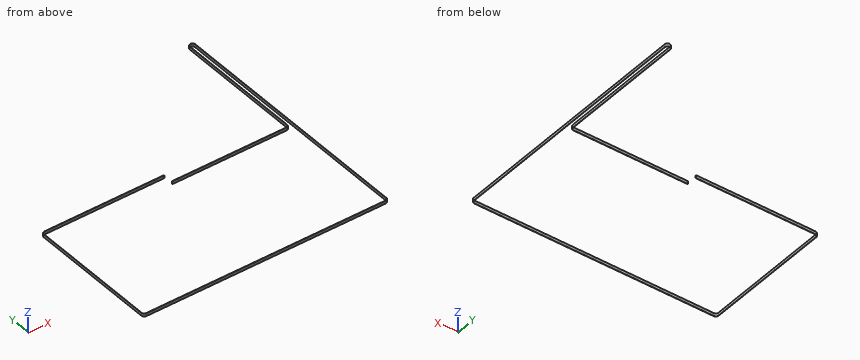
from build123d import *

# Parameters (mm, degrees)
F1_DEPTH = 6


with BuildPart() as f1:
    # F0 (on Top) → F1 (new body)
    with BuildSketch(Plane.XY):
        with BuildLine():
            ThreePointArc((244.655, 259.59), (249.75, 264.685), (254.845, 259.59))
            Line((254.845, 259.59), (254.845, -261.41))
            ThreePointArc((254.845, -261.41), (253.352709, -265.012709), (249.75, -266.505))
            Line((249.75, -266.505), (-249.75, -266.505))
            ThreePointArc((-249.75, -266.505), (-253.352709, -265.012709), (-254.845, -261.41))
            Line((-254.845, -261.41), (-254.845, 5.09))
            Line((-254.845, 5.09), (-255.475, 5.09))
            Line((-255.475, 5.09), (-255.475, -261.41))
            ThreePointArc((-255.475, -261.41), (-253.798186, -265.458186), (-249.75, -267.135))
            Line((-249.75, -267.135), (249.75, -267.135))
            ThreePointArc((249.75, -267.135), (253.798186, -265.458186), (255.475, -261.41))
            Line((255.475, -261.41), (255.475, 259.59))
            ThreePointArc((255.475, 259.59), (249.75, 265.315), (244.025, 259.59))
            Line((244.025, 259.59), (244.025, -5.09))
            ThreePointArc((244.025, -5.09), (242.532709, -8.692709), (238.93, -10.185))
            Line((238.93, -10.185), (0, -10.185))
            Line((0, -10.185), (0, -10.815))
            Line((0, -10.815), (238.93, -10.815))
            ThreePointArc((238.93, -10.815), (242.978186, -9.138186), (244.655, -5.09))
            Line((244.655, -5.09), (244.655, 259.59))
        make_face()
        with BuildLine():
            Line((-255.475, 5.09), (-254.845, 5.09))
            ThreePointArc((-254.845, 5.09), (-253.352709, 8.692709), (-249.75, 10.185))
            Line((-249.75, 10.185), (0, 10.185))
            Line((0, 10.185), (0, 10.815))
            Line((0, 10.815), (-249.75, 10.815))
            ThreePointArc((-249.75, 10.815), (-253.798186, 9.138186), (-255.475, 5.09))
        make_face()
    extrude(amount=F1_DEPTH)


solid = f1.part
Here's how the part is built. I have some questions about the finished solid (model axes, mm). Give positions to 0.01 mm unless a question says otherwise; leave off trailing zeros. Order: outer loops, then holes, each group sorted by start corner. A loop starts at its lowest first (then second) coordinate and runs counter-clockwise, first axis right, second up. Notation, with made-up numbers: (11, 49.5) -> (48, 49.5) arc R15 ccw to (48, 60.5) -> close; hole circle Ø6 at (-14.75, -2.5). An arc over 180 degrees is marked (long way). Use a Markdown table: item, result. Add a question column.
Item 1: Imagine slicing it at B-B on y = 59.5. Please give me the cut outline in (x, z) (3 decimals), plus the area to 3 significant figures.
Item 2: Imagine slicing it at C-C on z = 1.45. Please give me the cut outline in (x, y) (3 decimals).
Item 3: Imagine slicing it at A-A on x = 101. Please give me the cut outline in (y, z) (3 decimals), plus the area to 3 significant figures.
Item 4: Will these pins go through, and if not, where does the flat tip stop? pin 1 (1 mm diameter, centred on x = 178, z = 3, fed in from +Y) (3 decimals); pin 2 (2 mm diameter, centred on x = -186, z = 3, fed in from +Y) (3 decimals); pin 3 (1.8 mm diameter, centred on y = 64, z = 4, fed in from -X) (3 decimals).
Item 5: I need wall thicknesses on line 1 (X direction, y = -3, z = 3.4) (3 decimals); line 2 (X direction, y = 52, z = 1.05) (3 decimals); line 3 (Y direction, x = 104, z = 2.65) (3 decimals). Which ranges of each line are inside material? Lowest first, please.
Data:
| question | item | result |
|---|---|---|
| 1 | outline | (244.025, 0) -> (244.655, 0) -> (244.655, 6) -> (244.025, 6) -> close; (254.845, 0) -> (255.475, 0) -> (255.475, 6) -> (254.845, 6) -> close |
| 1 | area | 7.56 mm² |
| 2 | outline | (-255.475, -261.41) arc R5.725 ccw to (-249.75, -267.135) -> (249.75, -267.135) arc R5.725 ccw to (255.475, -261.41) -> (255.475, 259.59) arc R5.725 ccw to (244.025, 259.59) -> (244.025, -5.09) arc R5.095 cw to (238.93, -10.185) -> (0, -10.185) -> (0, -10.815) -> (238.93, -10.815) arc R5.725 ccw to (244.655, -5.09) -> (244.655, 259.59) arc R5.095 cw to (254.845, 259.59) -> (254.845, -261.41) arc R5.095 cw to (249.75, -266.505) -> (-249.75, -266.505) arc R5.095 cw to (-254.845, -261.41) -> (-254.845, 5.09) arc R5.095 cw to (-249.75, 10.185) -> (0, 10.185) -> (0, 10.815) -> (-249.75, 10.815) arc R5.725 ccw to (-255.475, 5.09) -> close |
| 3 | outline | (-267.135, 0) -> (-266.505, 0) -> (-266.505, 6) -> (-267.135, 6) -> close; (-10.815, 0) -> (-10.185, 0) -> (-10.185, 6) -> (-10.815, 6) -> close |
| 3 | area | 7.56 mm² |
| 4 | pin 1 | stops at y = -10.185 |
| 4 | pin 2 | stops at y = 10.815 |
| 4 | pin 3 | stops at x = 244.025 |
| 5 | line 1 | x = -255.475 to -254.845, 244.025 to 244.655, 254.845 to 255.475 |
| 5 | line 2 | x = 244.025 to 244.655, 254.845 to 255.475 |
| 5 | line 3 | y = -267.135 to -266.505, -10.815 to -10.185 |
